Autodesk Inventor part; units mm, degrees
ref_plane "YZ Plane" through (0, 0, 0) normal (1, 0, 0) x (0, 1, 0)
ref_plane "XZ Plane" through (0, 0, 0) normal (0, 1, 0) x (-1, 0, 0)
ref_plane "XY Plane" through (0, 0, 0) normal (0, 0, 1) x (1, 0, 0)
sketch "Sketch1" plane through (0, 0, 0) normal (0, 0, 1) x (1, 0, 0)
  line L0 (-30, 44) -> (-30, -44)
  line L1 (-30, -44) -> (30, -44)
  line L2 (30, -44) -> (30, 44)
  line L3 (30, 44) -> (-30, 44)
  circle A0 centre (22.5, -24) radius 3
  circle A1 centre (-22.5, -24) radius 3
  line L4 (-15, -4) -> (-30, -4)
  line L5 (-30, -4) -> (-30, -44)
  line L6 (-15, -44) -> (-30, -44)
  line L7 (-15, -4) -> (-15, -44)
  circle A2 centre (-22.5, 24) radius 3
  line L8 (-15, 44) -> (-30, 44)
  line L9 (-30, 44) -> (-30, 4)
  line L10 (-15, 4) -> (-30, 4)
  line L11 (-15, 44) -> (-15, 4)
  circle A3 centre (-22.5, 24) radius 3
  line L12 (-15, 4) -> (-30, 4)
  line L13 (-30, 4) -> (-30, 44)
  line L14 (-15, 44) -> (-30, 44)
  line L15 (-15, 4) -> (-15, 44)
  circle A4 centre (-22.5, 24) radius 3
  line L16 (-15, 4) -> (-30, 4)
  line L17 (-30, 4) -> (-30, 44)
  line L18 (-15, 44) -> (-30, 44)
  line L19 (-15, 4) -> (-15, 44)
  circle A5 centre (-22.5, 24) radius 3
  line L20 (-15, 4) -> (-30, 4)
  line L21 (-30, 4) -> (-30, 44)
  line L22 (-15, 44) -> (-30, 44)
  line L23 (-15, 4) -> (-15, 44)
  circle A6 centre (-22.5, 24) radius 3
  line L24 (-15, 4) -> (-30, 4)
  line L25 (-30, 4) -> (-30, 44)
  line L26 (-15, 44) -> (-30, 44)
  line L27 (-15, 4) -> (-15, 44)
  circle A7 centre (-22.5, 24) radius 3
  line L28 (-15, 4) -> (-30, 4)
  line L29 (-30, 4) -> (-30, 44)
  line L30 (-15, 44) -> (-30, 44)
  line L31 (-15, 4) -> (-15, 44)
  circle A8 centre (22.5, 24) radius 3
  line L32 (30, 4) -> (15, 4)
  line L33 (15, 4) -> (15, 44)
  line L34 (30, 44) -> (15, 44)
  line L35 (30, 4) -> (30, 44)
  point P0 (0, 0)
extrude "Extrusion1" add sketch "Sketch1" along normal blind 5
sketch "Sketch2" plane through (0, 0, 5) normal (0, 0, 1) x (1, 0, 0)
  line L0 (30, 44) -> (-30, 44)
  line L1 (-30, 44) -> (-30, -44)
  line L2 (30, 44) -> (-30, 44)
  line L3 (-30, 44) -> (-30, 32)
  line L4 (-30, 32) -> (30, 32)
  line L5 (30, 32) -> (30, 44)
  line L6 (30, -44) -> (-30, -44)
  line L7 (-30, -44) -> (-30, -32)
  line L8 (-30, -32) -> (30, -32)
  line L9 (30, -32) -> (30, -44)
  point P0 (0, 0)
  dimension "d2" = 12
  dimension "d3" = 12
extrude "Extrusion2" add sketch "Sketch2" along normal blind 40
sketch "Sketch3" plane through (0, 0, 45) normal (0, 0, 1) x (1, 0, 0)
  circle A0 centre (21, 38) radius 1.5
  circle A1 centre (-21, 38) radius 1.5
  circle A2 centre (21, -38) radius 1.5
  circle A3 centre (-21, -38) radius 1.5
  line L0 (-30, 32) -> (30, 32)
  line L1 (-30, -44) -> (30, -44)
  line L2 (30, 32) -> (30, 44)
  line L3 (30, -44) -> (30, -32)
  point P0 (0, 0)
  dimension "d6" = 3
  dimension "d7" = 3
  dimension "d8" = 3
  dimension "d9" = 3
  dimension "d10" = 6
  dimension "d11" = 6
  dimension "d12" = 42
  dimension "d13" = 42
  dimension "d14" = 9
  dimension "d15" = 9
extrude "Extrusion3" cut sketch "Sketch3" against normal blind 5
sketch "Sketch4" plane through (0, 0, 5) normal (0, 0, 1) x (1, 0, 0)
  circle A0 centre (22.5, 24) radius 3
  circle A1 centre (22.5, 24) radius 3.5
  circle A2 centre (22.5, -24) radius 3
  circle A3 centre (22.5, -24) radius 3.5
  circle A4 centre (-22.5, 24) radius 3
  circle A5 centre (-22.5, 24) radius 3.5
  circle A6 centre (-22.5, -24) radius 3
  circle A7 centre (-22.5, -24) radius 3.5
  point P0 (0, 0)
  dimension "d18" = 7
  dimension "d19" = 7
  dimension "d20" = 7
  dimension "d21" = 7
extrude "Extrusion4" cut sketch "Sketch4" against normal blind 5 contours A0 | A1 | A2 | A3 | A4 | A5 | A6 | A7
ref_plane "Work Plane1" through (0, -44, 0) normal (-1, 0, 0) x (0, 0, 1)
sketch "Sketch5" plane through (0, -44, 0) normal (-1, 0, 0) x (0, 0, 1)
  line L0 (5, 76) -> (5, 12)
  line L1 (5, 76) -> (5, 51)
  line L2 (45, 76) -> (45, 88)
  line L3 (5, 51) -> (45, 76)
  line L4 (5, 76) -> (45, 76)
  line L5 (45, 76) -> (5, 76)
  line L6 (5, 12) -> (45, 12)
  line L7 (5, 12) -> (5, 37)
  line L8 (45, 12) -> (45, 0)
  line L9 (5, 37) -> (45, 12)
  line L10 (45, 12) -> (5, 12)
  point P0 (0, 44)
  dimension "d24" = 25
  dimension "d25" = 25
extrude "Extrusion5" add sketch "Sketch5" along normal mid plane 12
properties part number "bearingV2"
Input: part model. Units: mm. Frame: model coordinates. A direction names the side the tool comes from. Round coordinates to 2 decimals unless told otherwise and drop trailing zeros. Order: outer loops, then holes, each group sorted by start corner. A loop starts at its lowest first (then second) coordinate and runs counter-clockwise, first axis right, second up. Notation, with made-up numbers: (62.25, 7.5) - (80.25, 7.5) arc R29 cw to (80.25, 39.5) - close; hole circle Ø8 at (51.5, 15). An arc over 180 degrees is marked (long way). Answer as a JSON object with one key per item and string values. Group by question number.
(1) Cut plane C-C (x = 15). Return loops of the section in (y, z).
(2) Cut plane A-A (y = 24). Return loops of the section in (x, z), then the cut area to 3 significant figures.
(3) Reachability of faces 1 (the face through (-21, 38, 40)), 2 (the face through (0, 38, 45)), 3 (the face through (-6, -25, 16)), 4 (the face through (0.084, -19.325, 24.72)) from +Z, -Z, +X, -X, +Y, -Y: full face, straight path, thin tool, end or side. Return the list, or none.
(4) Cut plane B-B (z = 38). Return loops of the section in (x, y) (3 decimals), then the cut area to 4 significant figures.
(5) Draft query along X for faces 5 (the face through (24.38, -21.05, 2.54)), 6 (the face through (-6, 22, 20)), 7 (the face through (18, -32, 25)), 8 (the face through (25.84, 25.05, 2.54)). Return one class per face: released by +X, released by -X, zero draft, split by the parting line, or undercut.
(6) Cut plane D-D (y = -30). Return loops of the section in (x, z).
(7) Material intervals for probe 1 along Y at (x, z) = (-21, 42.35); probe 2 along Y at (x, z) = (-27, 41); probe 3 along Y at (x, z) = (-25, 4), sorted ascending. Write a range as from..to.
(8) Pin query (flat end, axial travel): P1, Ø0.9, axis at x = 21, y = -38.5, coming from the +Z side; P2, Ø7.5, axis at y = -23.5, z = 25, coming from the +X side; P3, Ø2, axis at x = 23, y = 5.5, coming from the +Z side; P4, Ø4, axis at x = 21, y = 38, coming from the +Z side. Return the tip coordinate at first contact, or that it passes through.
Here are the results:
{
 "1": {"outline": "(-44, 0) - (44, 0) - (44, 45) - (32, 45) - (32, 5) - (-32, 5) - (-32, 45) - (-44, 45) - close"},
 "2": {"outline": "(-30, 0) - (-26, 0) - (-26, 5) - (-30, 5) - close; (-19, 0) - (19, 0) - (19, 5) - (6, 5) - (6, 32.2) - (-6, 32.2) - (-6, 5) - (-19, 5) - close; (26, 0) - (30, 0) - (30, 5) - (26, 5) - close", "area": "556 mm^2"},
 "3": {"face 1": "+Z", "face 2": "+Z, +X, -X, +Y, -Y", "face 3": "+Z, -X", "face 4": "+Z, +X, -X"},
 "4": {"outline": "(-30, -44) - (30, -44) - (30, -32) - (6, -32) - (6, -27.625) - (-6, -27.625) - (-6, -32) - (-30, -32) - close; (-30, 32) - (-6, 32) - (-6, 27.625) - (6, 27.625) - (6, 32) - (30, 32) - (30, 44) - (-30, 44) - close", "area": "1,545 mm^2"},
 "5": {"face 5": "undercut", "face 6": "released by -X", "face 7": "zero draft", "face 8": "undercut"},
 "6": {"outline": "(-30, 0) - (30, 0) - (30, 5) - (6, 5) - (6, 41.8) - (-6, 41.8) - (-6, 5) - (-30, 5) - close"},
 "7": {"probe 1": "y = -44..-39.5, -36.5..-32, 32..36.5, 39.5..44", "probe 2": "y = -44..-32, 32..44", "probe 3": "y = -44..-26.45, -21.55..21.55, 26.45..44"},
 "8": {"P1": "stops at z = 40", "P2": "stops at x = 6", "P3": "stops at z = 5", "P4": "stops at z = 45"}
}
